Check sheet for the modelled part. Datum: model origin and axes. Units: mm. A direction names the side the tool comes from. Round coordinates to 2 decimals unless told otherwise and drop trailing zeros. Write each loop counter-clockwise with the first axis right and the second up, starting at its lowest first coordinate (ties: lowest second). Pieces come first, ordered by that corner, then holes. Notation, with made-up numbers: M -17.5,-4.75 L 22.5,-4.75 A23 ccw 22.5,28.25 Z; hole C 43,67.25 d1. An arc over 180 degrees is marked long. Answer in a Markdown table with one row per item.
```python
from build123d import *

# Parameters (mm, degrees)
SKETCH1_R           = 35
BOSS_EXTRUDE1_DEPTH = 10
SKETCH2_R           = 1.75
CUT_EXTRUDE1_DEPTH  = 51.497524692
SKETCH4_R           = 18.5
CUT_EXTRUDE2_DEPTH  = 7
SKETCH5_R           = 14
CUT_EXTRUDE3_DEPTH  = 51.497524692
FILLET1_R           = 0.5


with BuildPart() as part:
    # Sketch1 → Boss-Extrude1 (new body)
    with BuildSketch(Plane(origin=(0, 0, 0), x_dir=(1, 0, 0), z_dir=(0, 1, 0))):
        with Locations(Location((0, 0, 0), (0, 0, 270))):
            Circle(SKETCH1_R)
    extrude(amount=BOSS_EXTRUDE1_DEPTH)

    # Sketch2 → Cut-Extrude1 (cut, through all)
    with BuildSketch(Plane(origin=(0, 10, 0), x_dir=(1, 0, 0), z_dir=(0, 1, 0))):
        with Locations(Location((0, 32.5, 0), (0, 0, 270))):
            Circle(SKETCH2_R)
        with Locations(Location((32.5, 0, 0), (0, 0, 270))):
            Circle(SKETCH2_R)
        with Locations(Location((0, -32.5, 0), (0, 0, 270))):
            Circle(SKETCH2_R)
        with Locations(Location((-32.5, 0, 0), (0, 0, 270))):
            Circle(SKETCH2_R)
    extrude(amount=-CUT_EXTRUDE1_DEPTH, mode=Mode.SUBTRACT)

    # Sketch4 → Cut-Extrude2 (cut)
    with BuildSketch(Plane.XZ):
        with Locations(Location((0, 0, 0), (0, 0, 270))):
            Circle(SKETCH4_R)
    extrude(amount=-CUT_EXTRUDE2_DEPTH, mode=Mode.SUBTRACT)

    # Sketch5 → Cut-Extrude3 (cut, through all)
    with BuildSketch(Plane(origin=(0, 10, 0), x_dir=(1, 0, 0), z_dir=(0, 1, 0))):
        with Locations(Location((0, 0, 0), (0, 0, 270))):
            Circle(SKETCH5_R)
    extrude(amount=-CUT_EXTRUDE3_DEPTH, mode=Mode.SUBTRACT)

    # Fillet1
    fillet1_edges = [part.edges().sort_by_distance(p)[0] for p in [
        (0, 10, -35),
    ]]
    fillet(fillet1_edges, radius=FILLET1_R)


solid = part.part
```
1. Section check C-C, the plane y = 5. Record the cut outline in (x, z).
Found:
| item | result |
|---|---|
| outline | C 0,0 d70; hole C -32.5,0 d3.5; hole C 0,0 d37; hole C 0,-32.5 d3.5; hole C 0,32.5 d3.5; hole C 32.5,0 d3.5 |
2. Section check B-B, the plane z = 0. Record the cut outline in (x, y).
Found:
| item | result |
|---|---|
| outline | M -35,0 L -34.25,0 L -34.25,10 L -34.5,10 A0.5 ccw -35,9.5 Z; M -30.75,0 L -18.5,0 L -18.5,7 L -14,7 L -14,10 L -30.75,10 Z; M 14,7 L 18.5,7 L 18.5,0 L 30.75,0 L 30.75,10 L 14,10 Z; M 34.25,0 L 35,0 L 35,9.5 A0.5 ccw 34.5,10 L 34.25,10 Z |
3. Access from +Z, -Z, +X, -X, +Y, -Y to the whole of each face (thin tool, end or side, straight path). Record for faces 1 (the face through (14, 7, 3)), 2 (the face through (0.08, 5.07, 30.75)).
Found:
| item | result |
|---|---|
| face 1 | -Y |
| face 2 | +Y, -Y |
4. Go/stop test with flat-tipped pins: pin 1 (1 mm diameter, centred on x = -4.5, y = 8.5, fed in from +Z); pin 2 (25 mm diameter, centred on x = 0, z = 0, fed in from +Y); pin 3 (1.5 mm diameter, centred on y = 8.5, z = -22.5, fed in from +X); pin 4 (1 mm diameter, centred on y = 3.5, z = 9, fed in from +X). Record where each tip stops, or that it passes through.
Found:
| item | result |
|---|---|
| pin 1 | stops at z = 34.77 |
| pin 2 | passes through |
| pin 3 | stops at x = 27.42 |
| pin 4 | stops at x = 33.95 |
5. Section check A-A, the plane y = 8.5. Record the cut outline in (x, z).
Found:
| item | result |
|---|---|
| outline | C 0,0 d70; hole C -32.5,0 d3.5; hole C 0,0 d28; hole C 0,-32.5 d3.5; hole C 0,32.5 d3.5; hole C 32.5,0 d3.5 |
6. Draft check along Z on faces 3 (the face through (-21, 5, -28)), 4 (the face through (0.08, 5.07, -34.25)), 5 (the face through (-15, 10, 0)). Enter one of: +Z half, -Z half, draft (parallel to the pull), parting line (faces both ways), or undercut.
Found:
| item | result |
|---|---|
| face 3 | parting line |
| face 4 | undercut |
| face 5 | draft |
7. Scan lines: L1, parallel to X at y = 6.75, z = 0; L2, parallel to X at y = 9, z = 0; L3, parallel to Y at x = 5, z = 15.5. Record each from-to range of solid material in increasing order.
Found:
| item | result |
|---|---|
| L1 | x = -35 to -34.25, -30.75 to -18.5, 18.5 to 30.75, 34.25 to 35 |
| L2 | x = -35 to -34.25, -30.75 to -14, 14 to 30.75, 34.25 to 35 |
| L3 | y = 7 to 10 |
